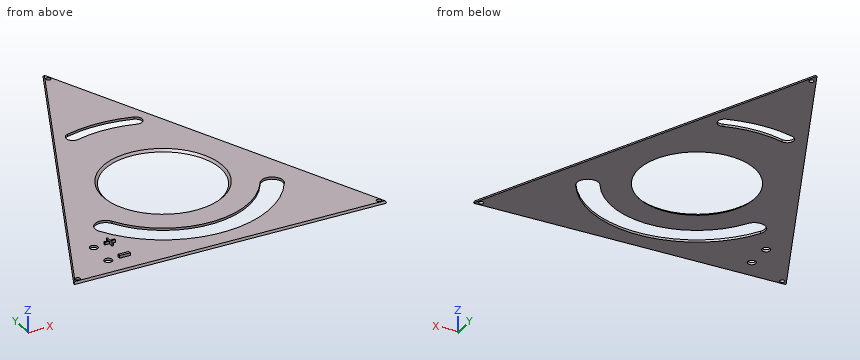
from build123d import *

# Parameters (mm, degrees)
BOSS_EXTRUDE1_DEPTH = 1.7
BOSS_EXTRUDE1_TAPER = 25
SKETCH2_R           = 40
CUT_EXTRUDE1_DEPTH  = 204.652444278
SKETCH3_R           = 1.75
CUT_EXTRUDE2_DEPTH  = 204.652444278
CHAMFER1_SIZE       = 5
CUT_EXTRUDE4_REACH  = 205.652
SKETCH4_R           = 3
SKETCH6_W           = 8
SKETCH6_H           = 2
BOSS_EXTRUDE2_DEPTH = 2


with BuildPart() as part:
    # Sketch1 → Boss-Extrude1 (new body)
    with BuildSketch(Plane.XY):
        Polygon((117.27472237, -93.523470279), (0, 166.487439626), (-117.27472237, -93.523470279), align=None)
    extrude(amount=BOSS_EXTRUDE1_DEPTH, taper=BOSS_EXTRUDE1_TAPER)

    # Sketch2 → Cut-Extrude1 (cut, through all)
    with BuildSketch(Plane.XY.offset(1.7)):
        Circle(SKETCH2_R)
    extrude(amount=-CUT_EXTRUDE1_DEPTH, mode=Mode.SUBTRACT)

    # Sketch3 → Cut-Extrude2 (cut, through all)
    with BuildSketch(Plane.XY.offset(1.7)):
        with Locations((0, 158.987439626)):
            Circle(SKETCH3_R)
        with Locations((112.77472237, -90.523470279)):
            Circle(SKETCH3_R)
        with Locations((-112.77472237, -90.523470279)):
            Circle(SKETCH3_R)
    extrude(amount=-CUT_EXTRUDE2_DEPTH, mode=Mode.SUBTRACT)

    # Chamfer1
    # the kernel refuses this chamfer: 5 mm, written as the material it takes off along each edge
    with BuildSketch(Plane(origin=(0, 0, 1.7), x_dir=(1, 0, 0), z_dir=(0, -1, 0))) as chamfer1_piece_1:
        Polygon((40, -CHAMFER1_SIZE), (40 + CHAMFER1_SIZE, 0), (40, 0), align=None)
    revolve(axis=Axis((0, 0, 1.7), (0, 0, 1)), mode=Mode.SUBTRACT)

    # Sketch4 → Cut-Extrude4 (cut, up to next)
    with BuildSketch(Plane.XY.offset(1.7), mode=Mode.PRIVATE) as cut_extrude4_sk1:
        with Locations((-83.047547857, -57.73074726)):
            Circle(SKETCH4_R)
    cut_extrude4_tool1 = extrude(cut_extrude4_sk1.sketch, amount=-CUT_EXTRUDE4_REACH, mode=Mode.PRIVATE) & part.part
    # Sketch4 → Cut-Extrude4 (cut, up to next)
    with BuildSketch(Plane.XY.offset(1.7), mode=Mode.PRIVATE) as cut_extrude4_sk2:
        with Locations((-83.047547857, -77.73074726)):
            Circle(SKETCH4_R)
    cut_extrude4_tool2 = extrude(cut_extrude4_sk2.sketch, amount=-CUT_EXTRUDE4_REACH, mode=Mode.PRIVATE) & part.part
    # Sketch4 → Cut-Extrude4 (cut, up to next)
    with BuildSketch(Plane.XY.offset(1.7), mode=Mode.PRIVATE) as cut_extrude4_sk3:
        with BuildLine():
            ThreePointArc((69.282032303, -40), (0, -80), (-69.282032303, -40))
            ThreePointArc((-69.282032303, -40), (-66.353829072, -29.07179677), (-55.425625842, -32))
            ThreePointArc((-55.425625842, -32), (0, -64), (55.425625842, -32))
            ThreePointArc((55.425625842, -32), (66.353829072, -29.07179677), (69.282032303, -40))
        make_face()
    cut_extrude4_tool3 = extrude(cut_extrude4_sk3.sketch, amount=-CUT_EXTRUDE4_REACH, mode=Mode.PRIVATE) & part.part
    # Sketch4 → Cut-Extrude4 (cut, up to next)
    with BuildSketch(Plane.XY.offset(1.7), mode=Mode.PRIVATE) as cut_extrude4_sk4:
        with BuildLine():
            ThreePointArc((-24.807362024, 86.513552634), (0, 90), (24.807362024, 86.513552634))
            ThreePointArc((24.807362024, 86.513552634), (28.235483724, 80.329057376), (22.050988465, 76.900935675))
            ThreePointArc((22.050988465, 76.900935675), (0, 80), (-22.050988465, 76.900935675))
            ThreePointArc((-22.050988465, 76.900935675), (-28.235483724, 80.329057376), (-24.807362024, 86.513552634))
        make_face()
    cut_extrude4_tool4 = extrude(cut_extrude4_sk4.sketch, amount=-CUT_EXTRUDE4_REACH, mode=Mode.PRIVATE) & part.part
    add(cut_extrude4_tool1.solids().sort_by_distance((-83.047548, -57.730747, 1.7))[0], mode=Mode.SUBTRACT)
    add(cut_extrude4_tool2.solids().sort_by_distance((-83.047548, -77.730747, 1.7))[0], mode=Mode.SUBTRACT)
    add(cut_extrude4_tool3.solids().sort_by_distance((0, -78.499912, 1.7))[0], mode=Mode.SUBTRACT)
    add(cut_extrude4_tool4.solids().sort_by_distance((0, 83.588343, 1.7))[0], mode=Mode.SUBTRACT)

    # Sketch6 → Boss-Extrude2 (add)
    with BuildSketch(Plane.XY.offset(1.7)):
        Polygon((-71.547547857, -53.73074726), (-70.547547857, -53.73074726), (-70.547547857, -57.23074726), (-67.047547857, -57.23074726), (-67.047547857, -58.23074726), (-70.547547857, -58.23074726), (-70.547547857, -61.73074726), (-71.547547857, -61.73074726), (-71.547547857, -58.23074726), (-75.047547857, -58.23074726), (-75.047547857, -57.23074726), (-71.547547857, -57.23074726), align=None)
        with Locations((-71.047547857, -77.73074726)):
            Rectangle(SKETCH6_W, SKETCH6_H)
    extrude(amount=BOSS_EXTRUDE2_DEPTH)


solid = part.part
The listing builds one solid part. Answer for the finished solid, in the listing's coordinates (mm). Round coordinates to 2 decimals unless told otherwise and drop trailing zeros. Write each loop counter-clockwise with the first axis right and the second up, starting at its lowest first coordinate (ties: lowest second). Pieces come first, ordered by that corner, then holes. Notation, with made-up numbers: M -18.5,87.25 L 24.5,87.25 A20 ccw 24.5,113.25 Z; hole C 17,0 d7. An arc over 180 degrees is marked long. Write each question's results on one line, items separated by ' | '. Start each with the question number.
Item 1: A cutting plane is placed at B-B on y = 0. Write down the section's boundary in (x, z), and give its area (3 significant figures).
Item 2: Flat-ended cylindrical pins translate along their axes: pin 1 Ø1.6 at (x, z) = (-69, 3) entering from +Y; pin 2 Ø1.6 at (x, z) = (-70.5, 3) entering from -Y; pin 3 Ø1 at (y, z) = (-56, 2.5) entering from -X. Find the tip coordinate at first contact, or state that the pin passes through.
Item 3: A cutting plane is placed at C-C on x = 34. State how many separate pieces and enclosed holes the cut face has, and give its area (3 significant figures).
Item 4: A cutting plane is placed at A-A on z = 2.7. Write down the section's boundary in (x, y).
Item 5: Straight lines are drawn through the part: L1, parallel to Y at x = -69, z = 2.3; L2, parallel to Z at x = 80, y = -36; L3, parallel to X at y = 21, z = 1.15. For each, find the intervals that lie inside material, in ascending order. Write a range as [from, to].
Check sheet entries:
1) outline: M -75.09,0 L -43.3,0 L -45,1.7 L -74.22,1.7 Z; M 43.3,0 L 75.09,0 L 74.22,1.7 L 45,1.7 Z | area: 104 mm²
2) pin 1: y = -57.23 | pin 2: y = -78.73 | pin 3: x = -71.55
3) separate pieces: 3 | enclosed holes: 0 | area: 185 mm²
4) outline: M -75.05,-78.73 L -67.05,-78.73 L -67.05,-76.73 L -75.05,-76.73 Z; M -75.05,-58.23 L -71.55,-58.23 L -71.55,-61.73 L -70.55,-61.73 L -70.55,-58.23 L -67.05,-58.23 L -67.05,-57.23 L -70.55,-57.23 L -70.55,-53.73 L -71.55,-53.73 L -71.55,-57.23 L -75.05,-57.23 Z
5) L1: [-78.73, -76.73], [-58.23, -57.23] | L2: [0, 1.7] | L3: [-65.03, -39.18], [39.18, 65.03]
